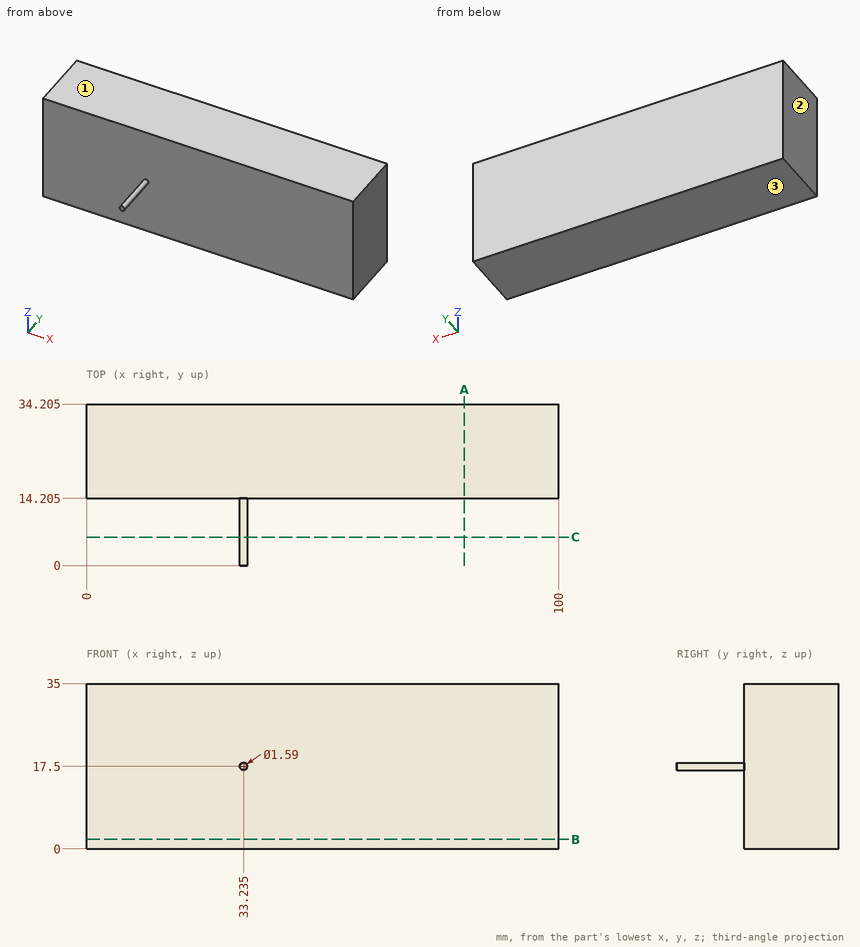
Input: dimensioned drawing with shaded views. Units: mm. Origin: part minimum x, y, z. Coordinates: 2 decimals unless noted, no trailing zeros. Write each loop counter-clockwise with the first axis right and the second up, starting at its lowest first coordinate (ties: lowest second). Pieces come first, ordered by that corner, then holes. Notation, with made-up numbers: M 51.25,60.25 L 70.25,60.25 A36 cw 70.25,96.25 Z; hole C 59.5,1.5 d1. An arc over 180 degrees is marked long. Answer as a JSON object with one key per item and string values. Group by question number.
(1) Section B-B on z = 2. Output: boundary loops of the cut face in (x, y) (3 decimals), plus the area to 3 significant figures.
(2) Section C-C on y = 6. Output: boundary loops of the cut face in (x, z) (3 decimals), plus the area to 3 significant figures.
(3) Mould query, pull axis Z, two halves, no side actions, for the marked faces 1, 2 and 3. Classes: pulls with the +Z half, pulls with the -Z half, needs draft (parallel to the pull), parting line crosses it, or undercut.
(4) Section A-A on x = 80. Output: boundary loops of the cut face in (y, z) (3 decimals).
(5) Contact query for a flat-ended pin moving along its axis: P1, Ø1.5, axis at x = 79, z = 4, coming from the -Y side (3 decimals). Output: stop coordinate, or through.
(6) Ray query, line 1 along Y through (x, z) = (74, 16) (3 decimals); line 2 along X through (y, z) = (12, 17). Return the intervals inside material, ascending. Write a range as [from, to].
Result set:
{
 "1": {"outline": "M 0,14.205 L 100,14.205 L 100,34.205 L 0,34.205 Z", "area": "2,000 mm2"},
 "2": {"outline": "C 33.235,17.5 d1.59", "area": "1.99 mm2"},
 "3": {"face 1": "pulls with the +Z half", "face 2": "needs draft", "face 3": "pulls with the -Z half"},
 "4": {"outline": "M 14.205,0 L 34.205,0 L 34.205,35 L 14.205,35 Z"},
 "5": {"P1": "stops at y = 14.205"},
 "6": {"line 1": "y = [14.205, 34.205]", "line 2": "x = [32.62, 33.85]"}
}
